from build123d import *

# Parameters (mm, degrees)
SKETCH_1_R          = 6.5
SKETCH_1_R_2        = 1.75
SKETCH_1_R_3        = 4.25
EXTRUDE_1_DEPTH     = 2
SKETCH_2_R          = 4.25
CUT_EXTRUDE_1_DEPTH = 3


with BuildPart() as part:
    # 草图1 → 凸台-拉伸1 (new body)
    with BuildSketch(Plane.XY):
        with BuildLine():
            Line((-6.617803136, 40.4809175), (-6.49997249, -0.018911091))
            ThreePointArc((-6.49997249, -0.018911091), (-0.009455556, 6.499993122), (6.5, 0))
            ThreePointArc((6.5, 0), (4.028885042, -5.100792617), (-1.505564714, -6.323232946))
            Line((-1.505564714, -6.323232946), (40.908736278, -16.422097799))
            ThreePointArc((40.908736278, -16.422097799), (36.882334136, -6.68604451), (47.389966762, -5.916431333))
            Line((47.389966762, -5.916431333), (4.857835124, 44.682262111))
            ThreePointArc((4.857835124, 44.682262111), (5.989207405, 42.725606264), (6.382169354, 40.499828591))
            ThreePointArc((6.382169354, 40.499828591), (-0.10837509, 33.999835469), (-6.617803136, 40.4809175))
        make_face()
        with Locations((-0.117830646, 40.499828591)):
            Circle(SKETCH_1_R)
        with Locations((-0.117830646, 40.499828591)):
            Circle(SKETCH_1_R_2, mode=Mode.SUBTRACT)
        with BuildLine():
            ThreePointArc((6.5, 0), (-0.009455556, 6.499993122), (-6.49997249, -0.018911091))
            ThreePointArc((-6.49997249, -0.018911091), (-5.094926397, -4.036300906), (-1.505564714, -6.323232946))
            ThreePointArc((-1.505564714, -6.323232946), (4.028885042, -5.100792617), (6.5, 0))
        make_face()
        Circle(SKETCH_1_R_3, mode=Mode.SUBTRACT)
        with Locations((42.414300993, -10.098864853)):
            Circle(SKETCH_1_R)
        with Locations((42.414300993, -10.098864853)):
            Circle(SKETCH_1_R_3, mode=Mode.SUBTRACT)
    extrude(amount=EXTRUDE_1_DEPTH)

    # 草图2 → 切除-拉伸1 (cut, through all)
    with BuildSketch(Plane.XY.offset(2)):
        with Locations((42.414300993, -10.098864853)):
            Circle(SKETCH_2_R)
        with BuildLine():
            Line((2.93856308, 36.863765144), (37.74927899, -4.549083802))
            Line((37.74927899, -4.549083802), (6.683866701, -2.079886036))
            ThreePointArc((6.683866701, -2.079886036), (5.358409291, 4.504159175), (-0.899681346, 6.941943062))
            Line((-0.899681346, 6.941943062), (2.93856308, 36.863765144))
        make_face()
    extrude(amount=-CUT_EXTRUDE_1_DEPTH, mode=Mode.SUBTRACT)


solid = part.part
The listing builds one solid part. Answer for the finished solid, in the listing's coordinates (mm). A direction names the side the tool comes from. Coordinates: 2 decimals unless noted, no trailing zeros. Order: outer loops, then holes, each group sorted by start corner. A loop starts at its lowest first (then second) coordinate and runs counter-clockwise, first axis right, second up. Notation, with made-up numbers: (2, 7) -> (24, 7) arc R22 ccw to (24, 39) -> close; hole circle Ø10 at (64.5, 85). An arc over 180 degrees is marked (long way). Answer in a Markdown table with one row per item. Add a question column.
Item 1: Find section A-A (y = 3.5). Write down the section's boundary in (x, z).
Item 2: Which of the six approach directions +Z, -Z, +X, -X, +Y, -Y give full straight-line access (tool end or side, diameter ignored) to faces 1 (the face through (0.993, 21.693, 1.014)), 2 (the face through (19.4, -11.3, 1))?
Item 3: Determine the mould class of faces 3 (the face through (20.1, 16.45, 1.01)), 4 (the face through (26.42, 19.03, 0.99)), 5 (the face through (23, 15, 0)) for opening direction Y: +Y half, -Y half, draft (parallel to the pull), parting line (faces both ways), or undercut.
Item 4: Find section B-B (y = 18). Write down the section's boundary in (x, z).
Item 5: Find the intervals of material crossed by L1, parallel to X at y = 3.5, z = 0.5; L2, parallel to X at y = 3, z = 0.85; L3, parallel to Y at x = 32.5, z = 0.5, in increasing order. Write a range as from..to.
Item 6: This flat-tipped pin is pushed along its axis until it touches: P1, Ø2, axis at x = -0.12, y = 40.5, coming from the -Z side. Where does it stop, or does it pass through?
Item 7: Find section C-C (z = 0.6). Write down the section's boundary in (x, y), then the cut area to 3 significant figures.
Item 8: Find section D-D (x = 16). Write down the section's boundary in (y, z).
Result set:
| question | item | result |
|---|---|---|
| 1 | outline | (-6.51, 0) -> (-2.41, 0) -> (-2.41, 2) -> (-6.51, 2) -> close; (2.41, 0) -> (6.06, 0) -> (6.06, 2) -> (2.41, 2) -> close; (30.98, 0) -> (39.47, 0) -> (39.47, 2) -> (30.98, 2) -> close |
| 2 | face 1 | +Z, -Z |
| 2 | face 2 | +Z, -Z, -X, -Y |
| 3 | face 3 | undercut |
| 3 | face 4 | +Y half |
| 3 | face 5 | draft |
| 4 | outline | (-6.55, 0) -> (0.52, 0) -> (0.52, 2) -> (-6.55, 2) -> close; (18.8, 0) -> (27.29, 0) -> (27.29, 2) -> (18.8, 2) -> close |
| 5 | L1 | x = -6.51..-2.41, 2.41..6.06, 30.98..39.47 |
| 5 | L2 | x = -6.51..-3.01, 3.01..6.32, 31.4..39.9 |
| 5 | L3 | y = -14.42..-4.13, 1.7..11.8 |
| 6 | P1 | passes through |
| 7 | outline | (-6.62, 40.48) -> (-6.5, -0.02) arc R6.5 ccw to (-1.51, -6.32) -> (40.91, -16.42) arc R6.5 ccw to (47.39, -5.92) -> (4.86, 44.68) arc R6.5 ccw to start; hole circle Ø8.5 at (0, 0); hole circle Ø3.5 at (-0.12, 40.5); hole (-0.9, 6.94) arc R7 cw to (6.68, -2.08) -> (37.75, -4.55) -> (2.94, 36.86) -> close; hole circle Ø8.5 at (42.41, -10.1) |
| 7 | area | 1,140 mm² |
| 8 | outline | (-10.49, 0) -> (-2.82, 0) -> (-2.82, 2) -> (-10.49, 2) -> close; (21.33, 0) -> (31.43, 0) -> (31.43, 2) -> (21.33, 2) -> close |
